Design review of the part built by this model. Coordinates are the model's own, in mm. Face numbers are marked on the shaded views. A direction names the side the tool comes from. Coordinates: 2 decimals unless noted, no trailing zeros. Write each loop counter-clockwise with the first axis right and the second up, starting at its lowest first coordinate (ties: lowest second). Pieces come first, ordered by that corner, then holes. Notation, with made-up numbers: (10.5, 15) - (53.5, 15) arc R27 cw to (53.5, 50) - close; hole circle Ø9 at (88, 79.5). An arc over 180 degrees is marked (long way). Use a Markdown table: item, result.
from build123d import *

# Parameters (mm, degrees)
F0_R     = 16.69467
F1_DEPTH = 127
F3_DEPTH = 136.144
F5_DEPTH = 107.696


with BuildPart() as f1:
    # F0 (on Front) → F1 (new body)
    with BuildSketch(Plane.XZ):
        Polygon((67.391418, 54.243322), (0, 54.243322), (-67.391418, 54.243322), (-67.391418, -66.123113), (0, -66.123113), (67.391418, -66.123113), align=None)
        Circle(F0_R, mode=Mode.SUBTRACT)
    extrude(amount=F1_DEPTH)

    # F2 (on face) → F3 (cut)
    with BuildSketch(Plane(origin=(-67.391418, 0, 0), x_dir=(0, -1, 0), z_dir=(-1, 0, 0))):
        Polygon((127, 54.243322), (40.401872, 54.243322), (127, -66.123113), align=None)
    extrude(amount=-F3_DEPTH, mode=Mode.SUBTRACT)

    # F4 (on face) → F5 (cut)
    with BuildSketch(Plane(origin=(-67.391418, 0, 0), x_dir=(0, -1, 0), z_dir=(-1, 0, 0))):
        Polygon((0, 54.243322), (0, 38.296405), (35.804231, 38.296405), (110.428944, -66.123113), (127, -66.123113), (40.401872, 54.243322), align=None)
    extrude(amount=-F5_DEPTH, mode=Mode.SUBTRACT)


solid = f1.part
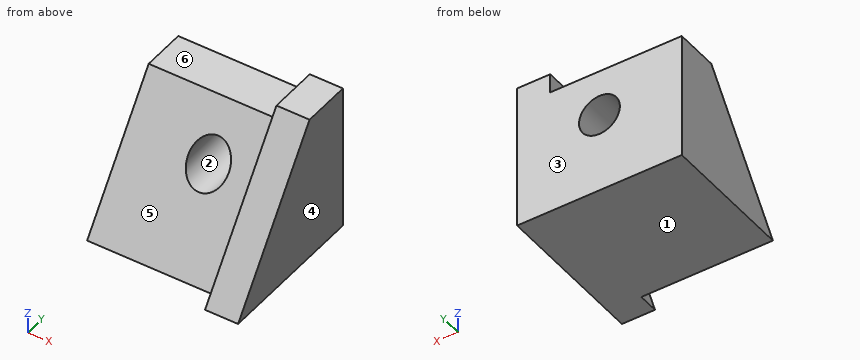
(1) Draft analysis for pull direction Z (two halves, no side actions). For the marked faces 1, 2 and 3, state which applies: +Z half, -Z half, draft (parallel to the pull), parting line (faces both ways), or undercut.
Determined:
| item | result |
|---|---|
| face 1 | -Z half |
| face 2 | undercut |
| face 3 | draft |
(2) Take a section at D-D on y = -59. Write out the cut boundary in (x, z).
Determined:
| item | result |
|---|---|
| outline | (-67.39, -66.12) - (67.39, -66.12) - (67.39, 28.39) - (40.3, 28.39) - (40.3, 5.84) - (15.64, 5.84) arc R16.69 cw (long way) to (-15.64, 5.84) - (-67.39, 5.84) - close |
(3) For L1, parallel to Z at x = 0, y = -28; L2, parallel to X at y = -59.5, z = 0; L3, parallel to Z at x = 24, y = -20.5, list the stretches that pass through material, from the lowest coordinate up. Write a range as from..to.
Determined:
| item | result |
|---|---|
| L1 | -66.12..-16.69, 16.69..38.3 |
| L2 | -67.39..-16.69, 16.69..67.39 |
| L3 | -66.12..38.3 |
(4) Take a section at B-B on y = -13.5. Write out the cut boundary in (x, z).
Determined:
| item | result |
|---|---|
| outline | (-67.39, -66.12) - (67.39, -66.12) - (67.39, 54.24) - (40.3, 54.24) - (40.3, 38.3) - (-67.39, 38.3) - close; hole circle Ø33.39 at (0, 0) |
(5) For pin 1 (3 mm diameter, centred on x = 30.5, z = 26, fed in from -Y); pin 2 (1.5 mm diameter, centred on x = 19.5, y = -68.5, fed in from +Z), all flat-tipped, find the tip position at first contact; note any pin that passes through.
Determined:
| item | result |
|---|---|
| pin 1 | y = -45.66 |
| pin 2 | z = -6.4 |
(6) Take a section at A-A on x = 8.5. Write out the cut boundary in (y, z), and give its area (3 significant figures).
Determined:
| item | result |
|---|---|
| outline | (-110.43, -66.12) - (0, -66.12) - (0, -14.37) - (-73.44, -14.37) - close; (-52.9, 14.37) - (0, 14.37) - (0, 38.3) - (-35.8, 38.3) - close |
| area | 5,820 mm2 |
(7) Machinability: for the marked faces 4, 5 and 6, which of the approach directions +Z, -Z, +X, -X, +Y, -Y give a long, thin tool a straight path to every point of the face, cutting with its end or side? Answer none if there is none.
Determined:
| item | result |
|---|---|
| face 4 | +Z, -Z, +X, +Y, -Y |
| face 5 | +Z, -X, -Y |
| face 6 | +Z, -X, +Y, -Y |
(8) Take a section at C-C on z = 0. Write out the cut boundary in (x, y).
Determined:
| item | result |
|---|---|
| outline | (-67.39, -63.17) - (-16.69, -63.17) - (-16.69, 0) - (-67.39, 0) - close; (16.69, -63.17) - (40.3, -63.17) - (40.3, -79.43) - (67.39, -79.43) - (67.39, 0) - (16.69, 0) - close |
